from build123d import *

# Parameters (mm, degrees)
F1_DEPTH = 1219.2


with BuildPart() as f1:
    # F0 (on Front) → F1 (new body)
    with BuildSketch(Plane.XZ):
        with BuildLine():
            ThreePointArc((101.6, 44.45), (99.740128, 48.940128), (95.25, 50.8))
            Line((95.25, 50.8), (-95.25, 50.8))
            ThreePointArc((-95.25, 50.8), (-99.740128, 48.940128), (-101.6, 44.45))
            Line((-101.6, 44.45), (-101.6, -44.45))
            ThreePointArc((-101.6, -44.45), (-99.740128, -48.940128), (-95.25, -50.8))
            Line((-95.25, -50.8), (95.25, -50.8))
            ThreePointArc((95.25, -50.8), (99.740128, -48.940128), (101.6, -44.45))
            Line((101.6, -44.45), (101.6, 44.45))
        make_face()
        with BuildLine():
            Line((-90.4875, 46.0375), (90.4875, 46.0375))
            ThreePointArc((90.4875, 46.0375), (94.977628, 44.177628), (96.8375, 39.6875))
            Line((96.8375, 39.6875), (96.8375, -39.6875))
            ThreePointArc((96.8375, -39.6875), (94.977628, -44.177628), (90.4875, -46.0375))
            Line((90.4875, -46.0375), (-90.4875, -46.0375))
            ThreePointArc((-90.4875, -46.0375), (-94.977628, -44.177628), (-96.8375, -39.6875))
            Line((-96.8375, -39.6875), (-96.8375, 39.6875))
            ThreePointArc((-96.8375, 39.6875), (-94.977628, 44.177628), (-90.4875, 46.0375))
        make_face(mode=Mode.SUBTRACT)
    extrude(amount=-F1_DEPTH)


solid = f1.part
Verification items for the finished model (mm, model axes). A direction names the side the tool comes from. Round coordinates to 2 decimals unless told otherwise and drop trailing zeros. Loops run counter-clockwise (first coordinate to the right, second up) from the corner with the lowest first, then second, coordinate; pieces in that order, holes last. Notation, with made-up numbers: (18, -38.75) - (44, -38.75) arc R29 cw to (44, -15.75) - close; hole circle Ø6 at (87, 66). An arc over 180 degrees is marked (long way). Answer in a Markdown table with one row per item. Add a question column.
Q1. Release check for a two-part mould opening along X. For faces 1 (the face through (101.6, 601, -1)), 2 (the face through (96.838, 601, 1)), 3 (the face through (-8, 1219.2, -49)) record: pulls with the +X half, pulls with the -X half, needs draft (parallel to the pull), parting line crosses it, or undercut.
Q2. Section check A-A on y = 1115. Enter the section's corners in (x, z), plus the area to 3 significant figures.
Q3. Tool access check on faces 4 (the face through (-96.838, 601, -1)), 5 (the face through (-101.6, 601, 1)). Record the directions out of +Z, -Z, +X, -X, +Y, -Y that give a thin tool (end or side, any length) a straight path to the whole face; none if there is none.
Q4. Section check B-B on z = 16. Enter the section's corners in (x, y), plus the area to 3 significant figures.
Q5. Section check C-C on x = 7. Enter the section's corners in (y, z).
Q6. Material ranges on line 1 (X direction, y = 419, z = -25); line 2 (Z direction, x = -88.5, y = 151); line 3 (X direction, y = 632, z = 43.5), recorded low to high.
Found:
| question | item | result |
|---|---|---|
| 1 | face 1 | pulls with the +X half |
| 1 | face 2 | undercut |
| 1 | face 3 | needs draft |
| 2 | outline | (-101.6, -44.45) arc R6.35 ccw to (-95.25, -50.8) - (95.25, -50.8) arc R6.35 ccw to (101.6, -44.45) - (101.6, 44.45) arc R6.35 ccw to (95.25, 50.8) - (-95.25, 50.8) arc R6.35 ccw to (-101.6, 44.45) - close; hole (-96.84, -39.69) arc R6.35 ccw to (-90.49, -46.04) - (90.49, -46.04) arc R6.35 ccw to (96.84, -39.69) - (96.84, 39.69) arc R6.35 ccw to (90.49, 46.04) - (-90.49, 46.04) arc R6.35 ccw to (-96.84, 39.69) - close |
| 2 | area | 2,810 mm² |
| 3 | face 4 | +Y, -Y |
| 3 | face 5 | +Z, -Z, -X, +Y, -Y |
| 4 | outline | (-101.6, 0) - (-96.84, 0) - (-96.84, 1219.2) - (-101.6, 1219.2) - close; (96.84, 0) - (101.6, 0) - (101.6, 1219.2) - (96.84, 1219.2) - close |
| 4 | area | 11,600 mm² |
| 5 | outline | (0, -50.8) - (1219.2, -50.8) - (1219.2, -46.04) - (0, -46.04) - close; (0, 46.04) - (1219.2, 46.04) - (1219.2, 50.8) - (0, 50.8) - close |
| 6 | line 1 | x = -101.6 to -96.84, 96.84 to 101.6 |
| 6 | line 2 | z = -50.8 to -46.04, 46.04 to 50.8 |
| 6 | line 3 | x = -101.6 to -95.57, 95.57 to 101.6 |
